from build123d import *

# Parameters (mm, degrees)
CHAMFER1_SIZE       = 0.8
CHAMFER2_SIZE       = 1
SKETCH3_W           = 14.289580605
SKETCH3_H           = 3
CUT_EXTRUDE1_DEPTH  = 1
SKETCH5_R           = 8.987407092
CUT_EXTRUDE3_DEPTH  = 8
BOSS_EXTRUDE1_DEPTH = 10
CHAMFER3_SIZE       = 0.5
CUT_EXTRUDE4_DEPTH  = 35


with BuildPart() as part:
    # Sketch1 → Revolve1 (revolve)
    with BuildSketch(Plane.XY, mode=Mode.PRIVATE) as revolve1_sk:
        Polygon((31, 0), (31, 5.75), (28.321868185, 5.75), (28.321868185, 5.5), (0, 5.5), (0, 0), align=None)
    revolve(revolve1_sk.sketch.rotate(Axis((0, 0, 0), (1, 0, 0)), 90), axis=Axis((0, 0, 0), (1, 0, 0)))

    # Chamfer1
    chamfer1_edges = [part.edges().sort_by_distance(p)[0] for p in [
        (31, 0, -5.75),
    ]]
    chamfer(chamfer1_edges, length=CHAMFER1_SIZE)

    # Chamfer2
    chamfer2_edges = [part.edges().sort_by_distance(p)[0] for p in [
        (0, 0, -5.5),
    ]]
    chamfer(chamfer2_edges, length=CHAMFER2_SIZE)

    # Sketch3 → Cut-Extrude1 (cut)
    with BuildSketch(Plane(origin=(31, 0, 0), x_dir=(0, 0, -1), z_dir=(1, 0, 0))):
        with Locations((-0.669103075, 0)):
            Rectangle(SKETCH3_W, SKETCH3_H)
    extrude(amount=-CUT_EXTRUDE1_DEPTH, mode=Mode.SUBTRACT)

    # Sketch5 → Cut-Extrude3 (cut)
    with BuildSketch(Plane.ZY):
        Circle(SKETCH5_R)
    extrude(amount=-CUT_EXTRUDE3_DEPTH, mode=Mode.SUBTRACT)

    # Sketch6 → Boss-Extrude1 (add)
    with BuildSketch(Plane.ZY.offset(-8)):
        with BuildLine():
            Line((-4.25, 3), (-4.25, -3))
            ThreePointArc((-4.25, -3), (0, -5), (4.25, -3))
            Line((4.25, -3), (4.25, 3))
            ThreePointArc((4.25, 3), (0, 5), (-4.25, 3))
        make_face()
    extrude(amount=BOSS_EXTRUDE1_DEPTH)

    # Chamfer3
    chamfer3_edges = [part.edges().sort_by_distance(p)[0] for p in [
        (-2, 5, 0),
        (-2, -5, 0),
    ]]
    chamfer(chamfer3_edges, length=CHAMFER3_SIZE)

    # Sketch7 → Cut-Extrude4 (cut)
    with BuildSketch(Plane(origin=(30, 0, 0), x_dir=(0, 0, -1), z_dir=(1, 0, 0))):
        with BuildLine():
            Line((2.009844577, 1), (-4.990155423, 1))
            ThreePointArc((-4.990155423, 1), (-5.089366478, 0), (-4.990155423, -1))
            Line((-4.990155423, -1), (2.009844577, -1))
            Line((2.009844577, -1), (2.009844577, 1))
        make_face()
    extrude(amount=-CUT_EXTRUDE4_DEPTH, mode=Mode.SUBTRACT)


solid = part.part
Here's how the part is built. I have some questions about the finished solid (model axes, mm). A direction names the side the tool comes from. Give positions to 0.01 mm unless a question says otherwise; leave off trailing zeros. Loops run counter-clockwise (first coordinate to the right, second up) from the corner with the lowest first, then second, coordinate; pieces in that order, holes last. Notation, with made-up numbers: (32.25, 29.25) -> (47.25, 29.25) arc R29 ccw to (47.25, 50.25) -> close; hole circle Ø10 at (12.5, 16). An arc over 180 degrees is marked (long way). Answer as a JSON object with one key per item and string values. Group by question number.
Item 1: Imagine slicing it at D-D on x = 27.5. Write out the boundary of the cut face in (y, z), then the cut area to 3 significant figures.
Item 2: Will these pins go through, and if not, where does the flat tip stop? pin 1 (2 mm diameter, centred on x = 4.5, y = -2, fed in from +Z); pin 2 (6.5 mm diameter, centred on x = 2.5, y = -1.5, fed in from -Z); pin 3 (2 mm diameter, centred on x = 12, y = 0.5, fed in from +Z).
Item 3: Imagine slicing it at B-B on y = 0. Write out the boundary of the cut face in (x, z).
Item 4: Imagine slicing it at C-C on x = 1. Write out the boundary of the cut face in (y, z), then the cut area to 3 significant figures.
Item 5: On a 3-axis mill with a long thin cutter (end or side, diameter ignored), from which of +Z, -Z, +X, -X, +Y, -Y can I reach the whole of each face in a straight line? I mean faces 1 (the cylindrical face through (3, 5, 0)), 2 (the flat face through (8, 0, -5)), 3 (the flat face through (3, 2, 4.25)). Say none if no direction works.
Item 6: Thinking about a two-plate mould opening in Y: for faces 4 (the cylindrical face through (3, -5, 0)), 5 (the flat face through (30.5, 1.5, 0.1)), 6 (the flat face through (31, 3, 0)), 7 (the cylindrical face through (19.15, 0.01, 5.09)), which applies, pulls with the +Y half, pulls with the -Y half, needs draft (parallel to the pull), parting line crosses it, or undercut?
Item 7: Imagine slicing it at A-A on z = 0. Write out the boundary of the cut face in (x, y).
Item 8: I need wall thicknesses on L1, parallel to Y at x = 7, z = 0; L2, parallel to X at y = -0.5, z = -4; L3, parallel to X at y = 0.5, z = -4.75. Which ranges of each line are inside material? Lowest first, please.
Answer list:
{
 "1": {"outline": "circle Ø11 at (0, 0); hole (-1, -2.01) -> (1, -2.01) -> (1, 4.99) arc R5.09 ccw to (-1, 4.99) -> close", "area": "80.9 mm2"},
 "2": {"pin 1": "stops at z = 4.25", "pin 2": "stops at z = -4.25", "pin 3": "stops at z = 5.5"},
 "3": {"outline": "(-2, -4.25) -> (8, -4.25) -> (8, -5.5) -> (28.32, -5.5) -> (28.32, -5.75) -> (30, -5.75) -> (30, -2.01) -> (-2, -2.01) -> close; (8, 5.09) -> (30, 5.09) -> (30, 5.75) -> (28.32, 5.75) -> (28.32, 5.5) -> (8, 5.5) -> close"},
 "4": {"outline": "(-3, -4.25) -> (3, -4.25) arc R5.52 ccw to (3, 4.25) -> (1, 4.25) -> (1, -2.01) -> (-1, -2.01) -> (-1, 4.25) -> (-3, 4.25) arc R5.52 ccw to start", "area": "62.1 mm2"},
 "5": {"face 1": "-X, +Y", "face 2": "-X", "face 3": "+Z, -X, +Y, -Y"},
 "6": {"face 4": "pulls with the -Y half", "face 5": "undercut", "face 6": "needs draft", "face 7": "undercut"},
 "7": {"outline": "(-2, -4.5) -> (-1.5, -5) -> (8, -5) -> (8, -5.5) -> (28.32, -5.5) -> (28.32, -5.75) -> (30.2, -5.75) -> (31, -4.95) -> (31, -1.5) -> (30, -1.5) -> (30, -1) -> (-2, -1) -> close; (-2, 1) -> (30, 1) -> (30, 1.5) -> (31, 1.5) -> (31, 4.95) -> (30.2, 5.75) -> (28.32, 5.75) -> (28.32, 5.5) -> (8, 5.5) -> (8, 5) -> (-1.5, 5) -> (-2, 4.5) -> close"},
 "8": {"L1": "y = -5 to -1, 1 to 5", "L2": "x = -2 to 30", "L3": "x = 8 to 30"}
}
